```python
from build123d import *

# Parameters (mm, degrees)
ESTRUSIONE_ESTRUSIONE1_DEPTH = 20
ESTRUSIONE_ESTRUSIONE2_DEPTH = 10
SCHIZZO4_R                   = 2.8
TAGLIO_ESTRUSIONE2_DEPTH     = 2.8
TAGLIO_ESTRUSIONE3_START     = -20
TAGLIO_ESTRUSIONE3_DEPTH     = 20
FORO_PER_VITE_M6_1_D         = 6.6


with BuildPart() as part:
    # Schizzo1 → Estrusione-Estrusione1 (new body)
    with BuildSketch(Plane(origin=(0, 0, 0), x_dir=(1, 0, 0), z_dir=(0, 1, 0))):
        with BuildLine():
            Line((0, -91.7), (0, -141.7))
            ThreePointArc((0, -141.7), (91.083004293, -108.54849759), (139.547258602, -24.605946775))
            Line((139.547258602, -24.605946775), (90.306870951, -15.923537892))
            ThreePointArc((90.306870951, -15.923537892), (81.799772383, -41.444990506), (66.252536018, -63.399459549))
            Line((66.252536018, -63.399459549), (50.931647156, -76.255211743))
            ThreePointArc((50.931647156, -76.255211743), (26.610966566, -87.753897112), (0, -91.7))
        make_face()
    extrude(amount=ESTRUSIONE_ESTRUSIONE1_DEPTH)

    # Schizzo2 → Estrusione-Estrusione2 (add)
    with BuildSketch(Plane(origin=(0, 20, 0), x_dir=(1, 0, 0), z_dir=(0, 1, 0))):
        with BuildLine():
            Line((0, -100), (0, -141.7))
            ThreePointArc((0, -141.7), (91.083004293, -108.54849759), (139.547258602, -24.605946775))
            Line((139.547258602, -24.605946775), (98.480775301, -17.364817767))
            ThreePointArc((98.480775301, -17.364817767), (64.278760969, -76.604444312), (0, -100))
        make_face()
    extrude(amount=ESTRUSIONE_ESTRUSIONE2_DEPTH)

    # Schizzo4 → Taglio-Estrusione2 (cut)
    with BuildSketch(Plane(origin=(58.592091587, 0, 69.827335646), x_dir=(-0.7660444431189816, 0, 0.6427876096865353), z_dir=(-0.6427876096865353, 0, -0.7660444431189817))):
        with Locations((0, 10)):
            Circle(SCHIZZO4_R)
    extrude(amount=-TAGLIO_ESTRUSIONE2_DEPTH, mode=Mode.SUBTRACT)

    # Schizzo5 → Taglio-Estrusione3 (cut)
    with BuildSketch(Plane(origin=(0, 30, 0), x_dir=(1, 0, 0), z_dir=(0, 1, 0)).offset(TAGLIO_ESTRUSIONE3_START)):
        with BuildLine():
            Line((0, -141.7), (0, -111.7))
            ThreePointArc((0, -111.7), (71.799376002, -85.567164296), (110.003026011, -19.396501445))
            Line((110.003026011, -19.396501445), (139.547258602, -24.605946775))
            ThreePointArc((139.547258602, -24.605946775), (91.083004293, -108.54849759), (0, -141.7))
        make_face()
    extrude(amount=TAGLIO_ESTRUSIONE3_DEPTH, mode=Mode.SUBTRACT)

    # Foro per Vite M6-1 (through all)
    with Locations(Plane(origin=(80.348451211, 10, 95.75555539), x_dir=(0, 0, 1), z_dir=(0, 1, 0))):
        with Locations((0, 0)):
            Hole(FORO_PER_VITE_M6_1_D / 2)


solid = part.part
```
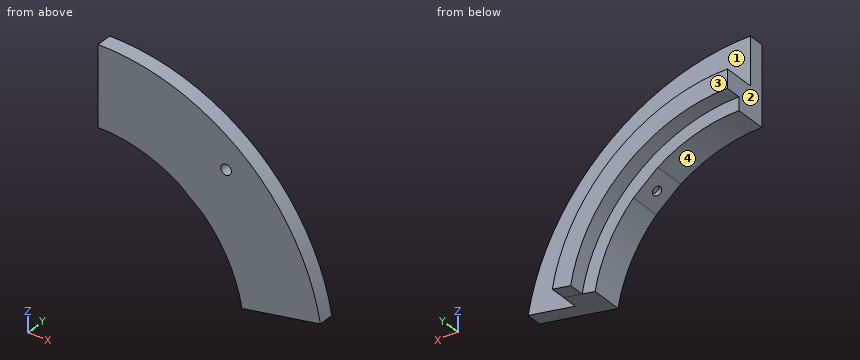
Could you check a few things on this model? Use its own coordinates, in mm. Face numbers are marked on the shaded views. A direction names the side the tool comes from. Coordinates: 2 decimals unless noted, no trailing zeros. Loops run counter-clockwise (first coordinate to the right, second up) from the corner with the lowest first, then second, coordinate; pieces in that order, holes last. Notation, with made-up numbers: M 64,21 L 106,21 A21 ccw 106,54 Z; hole C 12,58 d5. An arc over 180 degrees is marked long. Put each result on its own line as item: value. Start each with the question number.
(1) Suppose I cut it at A-A on y = 5.25. Please give me the cut outline in (x, z).
(2) Suppose I cut it at B-B on z = 45. Please give me the cut outline in (x, y), then the cut area to 3 significant figures.
(3) Thinking about a two-plate mould opening in X: for the marked faces 3 and 4, which applies, pulls with the +X half, pulls with the -X half, needs draft (parallel to the pull), parting line crosses it, or undercut?
(4) Suppose I cut it at D-D on y = 26.25. Please give me the cut outline in (x, z).
(5) Suppose I cut it at C-C on x = 25. Please give me the cut outline in (y, z), then the cut area to 3 significant figures.
(6) I need wall thicknesses on line 1 (Y direction, x = 21, z = 123); line 2 (Y direction, x = 85.5, z = 46); line 3 (X direction, y = 3.25, z = 93). Which ranges of each line are inside material? Lowest first, please. Write a range as from..to.
(7) For the marked faces 1 and 2, which set-ups out of +Z, -Z, +X, -X, +Y, -Y let a thin tool reach every point of the face, with its end or its side?
(8) Will these pins go through, and if not, where does the flat tip stop? P1, Ø10, axis at x = 82, y = 18.5, coming from the +Z side; P2, Ø25, axis at x = 67, z = 54.5, coming from the +Y side; P3, Ø4, axis at x = 23.5, y = 27, coming from the +Z side.
Solutions:
1. outline: M 0,91.7 A91.7 cw 50.93,76.26 L 66.25,63.4 A91.7 cw 90.31,15.92 L 139.55,24.61 A141.7 ccw 0,141.7 Z; hole C 80.35,95.76 d6.6
2. outline: M 79.9,0 L 134.36,0 L 134.36,10 L 102.23,10 L 102.23,30 L 89.3,30 L 89.3,20 L 79.9,20 Z
2. area: 897 mm2
3. face 3: needs draft
3. face 4: pulls with the -X half
4. outline: M 0,100 A100 cw 98.48,17.36 L 110,19.4 A111.7 ccw 0,111.7 Z
5. outline: M 0,88.23 L 20,88.23 L 20,96.82 L 30,96.82 L 30,108.87 L 10,108.87 L 10,139.48 L 0,139.48 Z
5. area: 839 mm2
6. line 1: y = 0..10
6. line 2: y = 0..20
6. line 3: x = 0..78.53, 82.16..106.91
7. face 1: +Z, +X, +Y
7. face 2: +Z, -Z, -X, +Y, -Y
8. P1: stops at z = 80.92
8. P2: stops at y = 20
8. P3: stops at z = 109.61
